The listing builds one solid part. Answer for the finished solid, in the listing's coordinates (mm). A direction names the side the tool comes from. Round coordinates to 2 decimals unless told otherwise and drop trailing zeros. Write each loop counter-clockwise with the first axis right and the second up, starting at its lowest first coordinate (ties: lowest second). Pieces come first, ordered by that corner, then holes.
(1) The mould has two halves that part along X. Classify faces 3 (the face through (-25, 24.388, 6)), 4 (the face through (-51.698, 12.844, 2.535)), 5 (the face through (25.576, 5, 10)), 6 (the face through (-49, 5, 5)): +X half, -X half, draft (parallel to the pull), parting line (faces both ways), or undercut.
(2) A cutting plane is placed at C-C, the plane x = 12. Give the vertices of the cut face in (y, z), and give its area (3 significant figures).
(3) For faces 1 (the face through (24, 4, 20)), 2 (the face through (-22.424, 5, 12)), determine the directions among +Z, -Z, +X, -X, +Y, -Y from which every point of the face is accessible in a straight line to the end or side of a thin tool.
(4) A cutting plane is placed at A-A, the plane z = 8.5. Give the vertices of the cut face in (x, y), and give its area (3 significant figures).
(5) Find the intervals of material crossed by probe 1 along X at (y, z) = (1.5, 7.5); probe 2 along X at (y, z) = (-8, 4.5); probe 3 along Z at (x, y) = (14.5, -2.5), in increasing order.
(6) Each of these flat-tipped pins is pushed along its axis until it touches: pin 1 Ø6 at (x, y) = (-43.5, -11) entering from +Z; pin 2 Ø5 at (x, y) = (-50.17, -6.68) entering from -Z. Where does it stop, or does it pass through?
(7) A cutting plane is placed at B-B, the plane y = -12. Give the vertices of the cut face in (x, z), and give its area (3 significant figures).
Autodesk Fusion 360 part; units mm, degrees
sketch "Sketch1" plane through (0, 0, 0) normal (0, 0, 1) x (1, 0, 0)
  line L0 (-74.4245, 24.3877) -> (25.5755, 24.3877)
  line L1 (25.5755, 24.3877) -> (25.5755, -15.6123)
  line L2 (25.5755, -15.6123) -> (-74.4245, -15.6123)
  line L3 (-74.4245, -15.6123) -> (-74.4245, 24.3877)
  dimension "d1" = 100
  dimension "d2" = 40
extrude "Extrude1" add sketch "Sketch1" along normal blind 5
sketch "Sketch2" plane through (0, 0, 5) normal (0, 0, 1) x (-1, 0, 0)
  line L0 (74.4245, 15.6123) -> (-25.5755, 15.6123)
  line L1 (-25.5755, 15.6123) -> (-25.5755, -24.3877)
  line L2 (-25.5755, -24.3877) -> (74.4245, -24.3877)
  line L3 (74.4245, -24.3877) -> (74.4245, 15.6123)
  line L4 (74.4245, -24.3877) -> (70.4245, -24.3877)
  line L5 (70.4245, -24.3877) -> (70.4245, 15.6123)
  line L6 (70.4245, 15.6123) -> (74.4245, 15.6123)
  line L7 (74.4245, 15.6123) -> (74.4245, -24.3877)
  line L8 (-25.5755, -24.3877) -> (-21.5755, -24.3877)
  line L9 (-21.5755, -24.3877) -> (-21.5755, 15.6123)
  line L10 (-21.5755, 15.6123) -> (-25.5755, 15.6123)
  line L11 (-25.5755, 15.6123) -> (-25.5755, -24.3877)
  line L12 (26.4245, -24.3877) -> (22.4245, -24.3877)
  line L13 (22.4245, -24.3877) -> (22.4245, 15.6123)
  line L14 (22.4245, 15.6123) -> (26.4245, 15.6123)
  line L15 (26.4245, 15.6123) -> (26.4245, -24.3877)
  point P0 (24.4245, -24.3877)
  dimension "d5" = 4
extrude "Extrude2" add sketch "Sketch2" along normal blind 15 contours L0 L2 L3 L4 L5 L6 L7 | L0 L2 L12 L13 L14 L15 | L0 L1 L2 L8 L9 L10 L11
sketch "Sketch3" plane through (0, 0, 5) normal (0, 0, 1) x (-1, 0, 0)
  line L0 (26.4245, 15.6123) -> (26.4245, -24.3877)
  line L1 (26.4245, -24.3877) -> (70.4245, -24.3877)
  line L2 (70.4245, -24.3877) -> (70.4245, 15.6123)
  line L3 (70.4245, 15.6123) -> (26.4245, 15.6123)
  circle A0 centre (50.1716, -13.3243) radius 1.6
  circle A1 centre (50.1716, 6.6757) radius 1.6
  circle A2 centre (0.1716, -13.3243) radius 1.6
  circle A3 centre (0.1716, 6.6757) radius 1.6
  point P0 (0.1716, -13.3243)
  point P1 (50.1716, 6.6757)
  point P2 (0.1716, 6.6757)
  dimension "d8" = 3.2
  dimension "d11" = -50
  dimension "d12" = 20
  dimension "d15" = 3.2
  dimension "d16" = 3.2
  dimension "d17" = 3.2
extrude "Extrude3" cut sketch "Sketch3" against normal blind 5 contours A0 | A1 | A2 | A3
Solutions:
1. face 3: draft
1. face 4: undercut
1. face 5: +X half
1. face 6: undercut
2. outline: (-15.61, 0) - (24.39, 0) - (24.39, 5) - (-15.61, 5) - close
2. area: 200 mm2
3. face 1: +Z, +X, -X, +Y, -Y
3. face 2: +Z, +Y, -Y
4. outline: (-74.42, -15.61) - (-70.42, -15.61) - (-70.42, 24.39) - (-74.42, 24.39) - close; (-26.42, -15.61) - (-22.42, -15.61) - (-22.42, 24.39) - (-26.42, 24.39) - close; (21.58, -15.61) - (25.58, -15.61) - (25.58, 24.39) - (21.58, 24.39) - close
4. area: 480 mm2
5. probe 1: x = -74.42 to -70.42, -26.42 to -22.42, 21.58 to 25.58
5. probe 2: x = -74.42 to -51.07, -49.27 to -1.07, 0.73 to 25.58
5. probe 3: z = 0 to 5
6. pin 1: stops at z = 5
6. pin 2: stops at z = 0
7. outline: (-74.42, 0) - (25.58, 0) - (25.58, 20) - (21.58, 20) - (21.58, 5) - (-22.42, 5) - (-22.42, 20) - (-26.42, 20) - (-26.42, 5) - (-70.42, 5) - (-70.42, 20) - (-74.42, 20) - close
7. area: 680 mm2
